Could you check a few things on this model? Use its own coordinates, in mm. Give positions to 0.01 mm unless a question says otherwise; leave off trailing zeros. Order: outer loops, then holes, each group sorted by start corner. A loop starts at its lowest first (then second) coordinate and runs counter-clockwise, first axis right, second up. Notation, with made-up numbers: M -0.5,-9.5 L 45.5,-9.5 A10 ccw 45.5,4.5 Z; hole C 24.25,-35.5 d3. An arc over 180 degrees is marked long. Use a Markdown table: item, result. Add a question column.
Item 1: If I drill on L1, parallel to Y at x = -7.75, z = 4.6; L2, parallel to Y at x = 9, z = 1; L3, parallel to Y at x = 6.75, z = 5, over which ranges is the centre line in solid material (lowest first)? Write a range as from..to.
Item 2: I'm going to push flat-ended pins straight in: pin 1 Ø1.8 at (y, z) = (-97.5, 4.5) entering from +X; pin 2 Ø2 at (x, z) = (8, 3.5) entering from +Y; pin 3 Ø3 at (y, z) = (-98, 3.5) entering from -X; pin 4 Ø1.4 at (x, y) = (-8, -41.15) entering from +Z. Where does each tip first touch, or does it pass through?
Item 3: Suppose I cut it at A-A on z = 3.5. Write out the boundary of the cut face in (x, y) (3 decimals), plus the area to 3 significant figures.
from build123d import *

# Parameters (mm, degrees)
ESQUISSE1_W             = 25
ESQUISSE1_H             = 200
BOSS_EXTRU_1_DEPTH      = 6
ESQUISSE2_R             = 1.175
ENL_V_MAT_EXTRU_1_DEPTH = 6
ESQUISSE3_W             = 7.5
ESQUISSE3_H             = 6
ENL_V_MAT_EXTRU_2_DEPTH = 6


with BuildPart() as part:
    # Esquisse1 → Boss.-Extru.1 (new body)
    with BuildSketch(Plane.XY):
        Rectangle(ESQUISSE1_W, ESQUISSE1_H)
    extrude(amount=BOSS_EXTRU_1_DEPTH)

    # Esquisse2 → Enlèv. mat.-Extru.1 (cut)
    with BuildSketch(Plane.XY.offset(6)):
        with Locations((8, -41.15)):
            Circle(ESQUISSE2_R)
        with Locations((-8, -41.15)):
            Circle(ESQUISSE2_R)
        with Locations((-8, -25.15)):
            Circle(ESQUISSE2_R)
        with Locations((8, -25.15)):
            Circle(ESQUISSE2_R)
    extrude(amount=-ENL_V_MAT_EXTRU_1_DEPTH, mode=Mode.SUBTRACT)

    # Esquisse3 → Enlèv. mat.-Extru.2 (cut)
    with BuildSketch(Plane.XY.offset(6)):
        with Locations((-8.75, -97)):
            Rectangle(ESQUISSE3_W, ESQUISSE3_H)
        with Locations((8.75, -97)):
            Rectangle(ESQUISSE3_W, ESQUISSE3_H)
        with Locations((8.75, 97)):
            Rectangle(ESQUISSE3_W, ESQUISSE3_H)
        with Locations((-8.75, 97)):
            Rectangle(ESQUISSE3_W, ESQUISSE3_H)
    extrude(amount=-ENL_V_MAT_EXTRU_2_DEPTH, mode=Mode.SUBTRACT)


solid = part.part
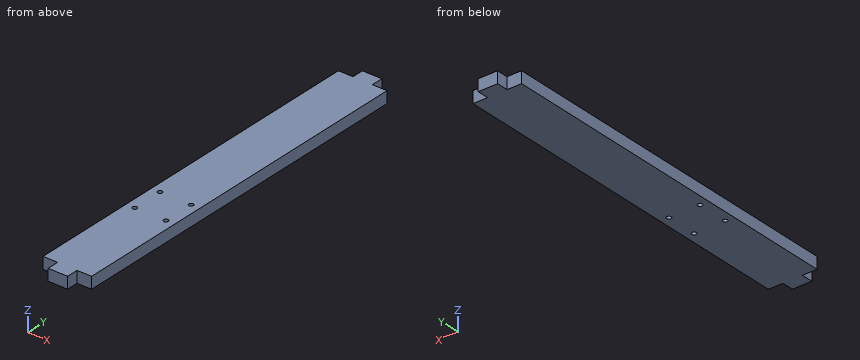
Findings below:
| question | item | result |
|---|---|---|
| 1 | L1 | y = -94..-42.3, -40..-26.3, -24..94 |
| 1 | L2 | y = -94..-41.77, -40.53..-25.77, -24.53..94 |
| 1 | L3 | y = -94..94 |
| 2 | pin 1 | stops at x = 5 |
| 2 | pin 2 | stops at y = 94 |
| 2 | pin 3 | stops at x = -5 |
| 2 | pin 4 | passes through |
| 3 | outline | M -12.5,-94 L -5,-94 L -5,-100 L 5,-100 L 5,-94 L 12.5,-94 L 12.5,94 L 5,94 L 5,100 L -5,100 L -5,94 L -12.5,94 Z; hole C -8,-41.15 d2.35; hole C -8,-25.15 d2.35; hole C 8,-41.15 d2.35; hole C 8,-25.15 d2.35 |
| 3 | area | 4,800 mm^2 |
